Geometry: final body of the model. Coordinates: model frame, mm. A direction names the side the tool comes from. Give positions to 0.01 mm unless a question says otherwise; leave off trailing zeros. Order: outer loops, then holes, each group sorted by start corner. A loop starts at its lowest first (then second) coordinate and runs counter-clockwise, first axis right, second up. Notation, with made-up numbers: (70.25, 32) - (89.25, 32) arc R23 cw to (89.25, 48) - close; hole circle Ø3 at (-16, 60.5). An arc over 180 degrees is marked (long way). One line per item, written item: value.
```python
from build123d import *

# Parameters (mm, degrees)
F1_DEPTH = 25
F2_R     = 10
F3_DEPTH = 1.9995178848
F5_R     = 10


with BuildPart() as f1:
    # F0 (on Front) → F1 (new body)
    with BuildSketch(Plane.XZ):
        with BuildLine():
            Line((-45, 25.9985178848), (-45, 24))
            Line((-45, 24), (0, 24))
            ThreePointArc((0, 24), (17.3205080757, 17.0277563773), (24.9799919936, 0))
            Line((24.9799919936, 0), (26.9799919936, 0))
            ThreePointArc((26.9799919936, 0), (18.7339457949, 18.4411739082), (0, 25.9985178848))
            Line((0, 25.9985178848), (-45, 25.9985178848))
        make_face()
    extrude(amount=F1_DEPTH)

    # F2 (on face) → F3 (cut, through all)
    with BuildSketch(Plane(origin=(0, 0, 24), x_dir=(1, 0, 0), z_dir=(0, 0, -1))):
        with Locations((-32, 12.5)):
            Circle(F2_R)
    extrude(amount=-F3_DEPTH, mode=Mode.SUBTRACT)

    # F4: F1 across plane


with BuildPart() as f1_1:
    add(f1.part)
    add(f1.part.mirror(Plane.XY))

    # F5
    f5_edges = [f1_1.edges().sort_by_distance(p)[0] for p in [
        (-45, -25, 24.999259),
        (-45, -25, -24.999259),
        (-45, 0, -24.999259),
        (-45, 0, 24.999259),
    ]]
    fillet(f5_edges, radius=F5_R)


solid = f1_1.part
```
1) Section A-A, the plane x = -5. Return loops of the section in (y, z).
Answers below:
outline: (-25, -26) - (0, -26) - (0, -24) - (-25, -24) - close; (-25, 24) - (0, 24) - (0, 26) - (-25, 26) - close
2) First-contact query: pin 1 (5 mm diameter, centred on x = 7, y = -13.5, fed in from -Z). Flat tip, straight axial feed; report the tip coordinate or a pass-through.
Answers below:
pin 1: z = -25.62
3) Mould query, pull axis Y, two halves, no side actions, for faces 1 (the face through (-34.17, -2.74, 24.99)), 2 (the face through (-41.99, -22.15, 24.99)), 3 (the face through (18.94, -12.32, 18.24)). Classes: released by +Y, released by -Y, zero draft, split by the parting line, or undercut.
Answers below:
face 1: undercut
face 2: released by -Y
face 3: zero draft
4) Section C-C, the plane x = -32. Return loops of the section in (y, z).
Answers below:
outline: (-25, -26) - (-22.5, -26) - (-22.5, -24) - (-25, -24) - close; (-25, 24) - (-22.5, 24) - (-22.5, 26) - (-25, 26) - close; (-2.5, -26) - (0, -26) - (0, -24) - (-2.5, -24) - close; (-2.5, 24) - (0, 24) - (0, 26) - (-2.5, 26) - close
5) Section D-D, the plane y = -4.5. Return loops of the section in (x, z), then the cut area to 3 significant figures.
Answers below:
outline: (-43.35, -26) - (-38, -26) - (-38, -24) - (-43.35, -24) - close; (-43.35, 24) - (-38, 24) - (-38, 26) - (-43.35, 26) - close; (-26, -26) - (0, -26) arc R27 ccw to (26.98, 0) arc R27 ccw to (0, 26) - (-26, 26) - (-26, 24) - (0, 24) arc R25 cw to (24.98, 0) arc R25 cw to (0, -24) - (-26, -24) - close
area: 285 mm^2
6) Material intervals for line 1 along Z through (x, y) = (-6, -5); line 2 along Y through (x, z) = (-32, -24.5); line 3 along Z through (x, y) = (20, -9.75), sorted ascending.
Answers below:
line 1: -26 to -24, 24 to 26
line 2: -25 to -22.5, -2.5 to 0
line 3: -17.14 to -14, 14 to 17.14
7) Set-up query: faces 4 (the face through (-42.15, -21.99, -24.99)), 5 (the face through (17.13, -12.32, -17.21)). Return all of +Z, -Z, +X, -X, +Y, -Y with unobstructed straight access to the full face (end or side cutting, diameter ignored); none if empty.
Answers below:
face 4: +Z, -Z, -X, -Y
face 5: -X, +Y, -Y
8) Section B-B, the plane y = -12.5. Return loops of the section in (x, z), then the cut area to 3 significant figures.
Answers below:
outline: (-45, -26) - (-42, -26) - (-42, -24) - (-45, -24) - close; (-45, 24) - (-42, 24) - (-42, 26) - (-45, 26) - close; (-22, -26) - (0, -26) arc R27 ccw to (26.98, 0) arc R27 ccw to (0, 26) - (-22, 26) - (-22, 24) - (0, 24) arc R25 cw to (24.98, 0) arc R25 cw to (0, -24) - (-22, -24) - close
area: 259 mm^2
